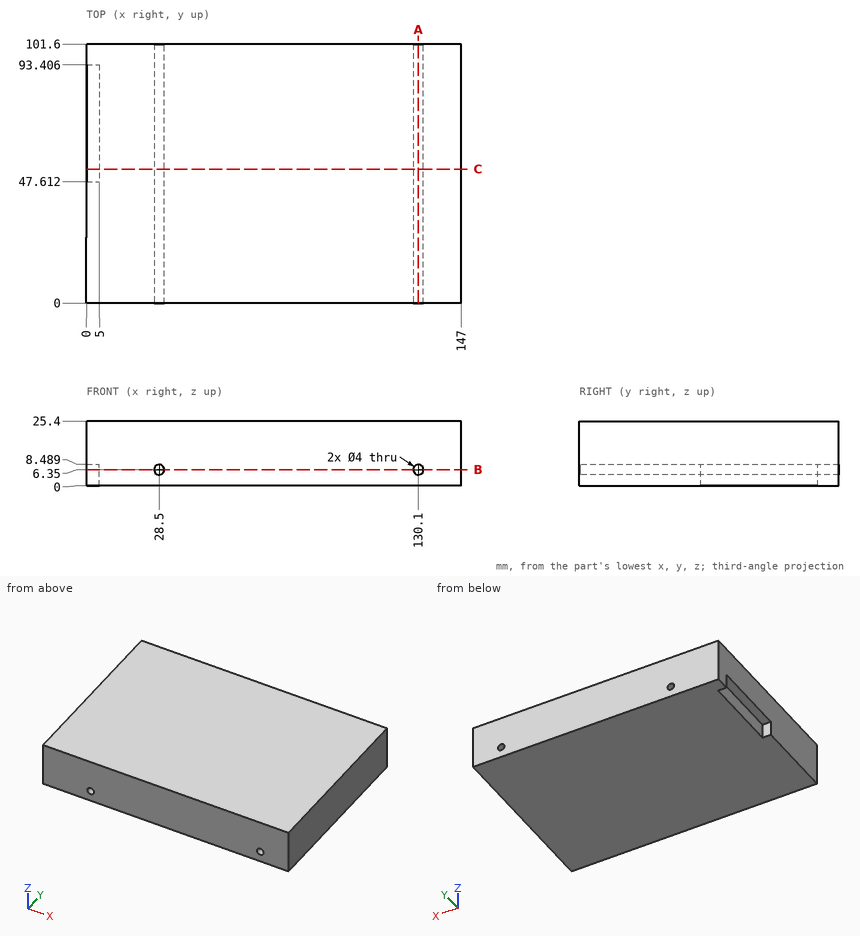
Can you work these out from the drawing? Everything is in mm from the part's minimum corner. Round coordinates to 2 decimals unless told otherwise and drop trailing zeros. Write each loop counter-clockwise with the first axis right and the second up, starting at its lowest first coordinate (ties: lowest second). Pieces come first, ordered by that corner, then holes. Notation, with made-up numbers: (40, 79) - (82, 79) arc R28 ccw to (82, 102) - close; hole circle Ø6 at (-34.75, 86.5). An arc over 180 degrees is marked (long way). Put each result on its own line as item: value. Start each with the question number.
(1) I need wall thicknesses on probe 1 along Z at (x, y) = (130, 43); probe 2 along X at (y, z) = (22.5, 5) (1 decimal). Which ranges of each line are inside material? Lowest first, please.
(2) I want a section at A-A, the plane x = 130.1. Please give me the cut outline in (y, z).
(3) I want a section at B-B, the plane z = 6.35. Please give me the cut outline in (x, y), plus the area to 3 significant figures.
(4) I want a section at C-C, the plane y = 52.5. Please give me the cut outline in (x, z), plus the area to 3 significant figures.
(5) Will this pin go through, and if not, where does the flat tip stop? pin 1 (5.5 mm diameter, centred on x = 2, y = 64.5, fed in from -Z).
Here are the results:
1. probe 1: z = 0 to 4.35, 8.35 to 25.4
1. probe 2: x = 0 to 27, 30 to 128.6, 131.6 to 147
2. outline: (0, 0) - (101.6, 0) - (101.6, 4.35) - (0, 4.35) - close; (0, 8.35) - (101.6, 8.35) - (101.6, 25.4) - (0, 25.4) - close
3. outline: (0, 0) - (26.5, 0) - (26.5, 101.6) - (0, 101.6) - (0, 93.41) - (5, 93.41) - (5, 47.61) - (0, 47.61) - close; (30.5, 0) - (128.1, 0) - (128.1, 101.6) - (30.5, 101.6) - close; (132.1, 0) - (147, 0) - (147, 101.6) - (132.1, 101.6) - close
3. area: 13,900 mm^2
4. outline: (0, 8.49) - (5, 8.49) - (5, 0) - (147, 0) - (147, 25.4) - (0, 25.4) - close; hole circle Ø4 at (28.5, 6.35); hole circle Ø4 at (130.1, 6.35)
4. area: 3,670 mm^2
5. pin 1: stops at z = 8.49
